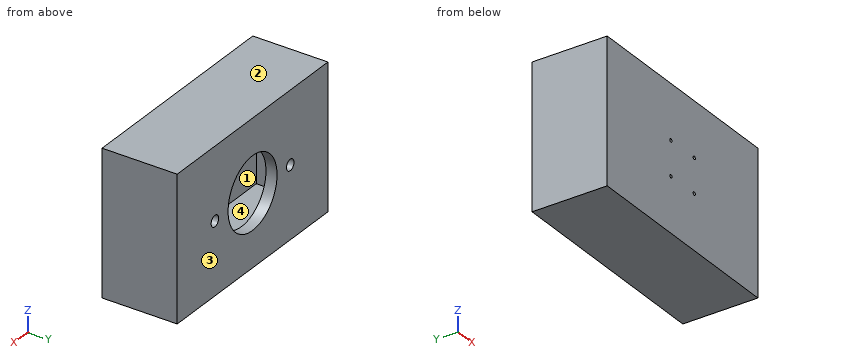
from build123d import *

# Parameters (mm, degrees)
SKETCH1_W           = 200
SKETCH1_H           = 130
BOSS_EXTRUDE1_DEPTH = 58
SHELL1_T            = -10
SKETCH2_R           = 1.5
CUT_EXTRUDE1_DEPTH  = 129.565158577
SKETCH3_W           = 200
SKETCH3_H           = 130
BOSS_EXTRUDE2_DEPTH = 10
CUT_EXTRUDE2_REACH  = 139.292
SKETCH4_R           = 32.5
SKETCH4_R_2         = 5


with BuildPart() as part:
    # Sketch1 → Boss-Extrude1 (new body)
    with BuildSketch(Plane(origin=(0, 0, 0), x_dir=(1, 0, 0), z_dir=(0, 1, 0))):
        Rectangle(SKETCH1_W, SKETCH1_H)
    extrude(amount=BOSS_EXTRUDE1_DEPTH)

    # Shell1
    shell1_openings = [part.faces().sort_by_distance(p)[0] for p in [
        (0, 58, 0),
    ]]
    offset(amount=SHELL1_T, openings=shell1_openings, kind=Kind.INTERSECTION)

    # Sketch2 → Cut-Extrude1 (cut, through all)
    with BuildSketch(Plane(origin=(0, 10, 0), x_dir=(1, 0, 0), z_dir=(0, 1, 0))):
        with Locations(Location((-15.5, 15.5, 0), (0, 0, 270))):
            Circle(SKETCH2_R)
        with Locations(Location((15.5, 15.5, 0), (0, 0, 270))):
            Circle(SKETCH2_R)
        with Locations(Location((-15.5, -15.5, 0), (0, 0, 270))):
            Circle(SKETCH2_R)
        with Locations(Location((15.5, -15.5, 0), (0, 0, 270))):
            Circle(SKETCH2_R)
    extrude(amount=-CUT_EXTRUDE1_DEPTH, mode=Mode.SUBTRACT)

    # Sketch3 → Boss-Extrude2 (add)
    with BuildSketch(Plane(origin=(0, 58, 0), x_dir=(1, 0, 0), z_dir=(0, 1, 0))):
        Rectangle(SKETCH3_W, SKETCH3_H)
    extrude(amount=BOSS_EXTRUDE2_DEPTH)

    # Sketch4 → Cut-Extrude2 (cut, up to next)
    with BuildSketch(Plane(origin=(0, 68, 0), x_dir=(1, 0, 0), z_dir=(0, 1, 0)), mode=Mode.PRIVATE) as cut_extrude2_sk1:
        with Locations(Location((0, 0, 0), (0, 0, 270))):
            Circle(SKETCH4_R)
    cut_extrude2_tool1 = extrude(cut_extrude2_sk1.sketch, amount=-CUT_EXTRUDE2_REACH, mode=Mode.PRIVATE) & part.part
    # Sketch4 → Cut-Extrude2 (cut, up to next)
    with BuildSketch(Plane(origin=(0, 68, 0), x_dir=(1, 0, 0), z_dir=(0, 1, 0)), mode=Mode.PRIVATE) as cut_extrude2_sk2:
        with Locations(Location((-50, 0, 0), (0, 0, 270))):
            Circle(SKETCH4_R_2)
    cut_extrude2_tool2 = extrude(cut_extrude2_sk2.sketch, amount=-CUT_EXTRUDE2_REACH, mode=Mode.PRIVATE) & part.part
    # Sketch4 → Cut-Extrude2 (cut, up to next)
    with BuildSketch(Plane(origin=(0, 68, 0), x_dir=(1, 0, 0), z_dir=(0, 1, 0)), mode=Mode.PRIVATE) as cut_extrude2_sk3:
        with Locations(Location((50, 0, 0), (0, 0, 270))):
            Circle(SKETCH4_R_2)
    cut_extrude2_tool3 = extrude(cut_extrude2_sk3.sketch, amount=-CUT_EXTRUDE2_REACH, mode=Mode.PRIVATE) & part.part
    add(cut_extrude2_tool1.solids().sort_by_distance((0, 68, 0))[0], mode=Mode.SUBTRACT)
    add(cut_extrude2_tool2.solids().sort_by_distance((-50, 68, 0))[0], mode=Mode.SUBTRACT)
    add(cut_extrude2_tool3.solids().sort_by_distance((50, 68, 0))[0], mode=Mode.SUBTRACT)


solid = part.part
Build history of the part. All positions in model axes, mm. Face numbers are marked on the shaded views. Round coordinates to 2 decimals unless told otherwise and drop trailing zeros. Loops run counter-clockwise (first coordinate to the right, second up) from the corner with the lowest first, then second, coordinate; pieces in that order, holes last. Notation, with made-up numbers: (-23, -40) -> (9, -40) arc R13 ccw to (9, -27) -> close; hole circle Ø1 at (25.25, 7.5). An arc over 180 degrees is marked (long way). One line per item, written item: value. Start each with the question number.
Q1. Two-plate mould, pull along Y, no slides. Class the marked faces 1, 2, 3 and 4: released by +Y, released by -Y, zero draft, split by the parting line, or undercut.
Q2. Cut at A-A on x = 70. List the corners of the cut face in (y, z).
Q3. Cut at B-B on z = 0. List the corners of the cut face in (x, y), plus the area to 3 significant figures.
Q4. Probe line 1 along X through (y, z) = (7.75, -15.5); line 2 along X through (y, z) = (64.75, 0); line 3 along Z through (x, y) = (8.5, 38). List the from-to ranges inside material, lowest first.
Q5. Cut at D-D on x = -50. List the corners of the cut face in (y, z).
Q6. Cut at C-C on y = 18. List the corners of the cut face in (x, z).
Q7. Drop a flat-ended pin along its axis: pin 1 Ø3.5 at (x, z) = (-15.5, -15.5) entering from +Y. Give the stop position or say it passes through.
Computed:
1. face 1: undercut
1. face 2: zero draft
1. face 3: released by +Y
1. face 4: undercut
2. outline: (0, -65) -> (68, -65) -> (68, 65) -> (0, 65) -> close; hole (10, -55) -> (58, -55) -> (58, 55) -> (10, 55) -> close
3. outline: (-100, 0) -> (100, 0) -> (100, 68) -> (55, 68) -> (55, 58) -> (90, 58) -> (90, 10) -> (-90, 10) -> (-90, 58) -> (-55, 58) -> (-55, 68) -> (-100, 68) -> close; (-45, 58) -> (-32.5, 58) -> (-32.5, 68) -> (-45, 68) -> close; (32.5, 58) -> (45, 58) -> (45, 68) -> (32.5, 68) -> close
3. area: 4,110 mm²
4. line 1: -100 to -17, -14 to 14, 17 to 100
4. line 2: -100 to -55, -45 to -32.5, 32.5 to 45, 55 to 100
4. line 3: -65 to -55, 55 to 65
5. outline: (0, -65) -> (68, -65) -> (68, -5) -> (58, -5) -> (58, -55) -> (10, -55) -> (10, 55) -> (58, 55) -> (58, 5) -> (68, 5) -> (68, 65) -> (0, 65) -> close
6. outline: (-100, -65) -> (100, -65) -> (100, 65) -> (-100, 65) -> close; hole (-90, -55) -> (90, -55) -> (90, 55) -> (-90, 55) -> close
7. pin 1: y = 10
